Design review of the part built by this model. Coordinates are the model's own, in mm. A direction names the side the tool comes from. Coordinates: 2 decimals unless noted, no trailing zeros. Loops run counter-clockwise (first coordinate to the right, second up) from the corner with the lowest first, then second, coordinate; pieces in that order, holes last. Notation, with made-up numbers: (-27.5, 72.25) -> (24.5, 72.25) arc R24 ccw to (24.5, 82.25) -> close; hole circle Ø9 at (-6, 88). An arc over 180 degrees is marked (long way). Use a Markdown table: item, result. Add a question column.
Q1. For probe 1 along Y at (x, z) = (7, 0.4); probe 2 along Y at (x, z) = (9.5, 0.95); probe 3 along X at (y, z) = (7.25, 1.8), list the stretches that pass through material, from the lowest coordinate up.
Q2. Take a section at A-A on x = 9.5. Write out the cut boundary in (y, z), plus the area to 3 significant figures.
Q3. For faces 1 (the face through (11, 4, 1)), 2 (the face through (-4, 9, 1)), 3 (the face through (10, -7, 1)), 4 (the face through (8.95, 5.03, 1.08)), list the 3-axis set-ups (+Z, -Z, +X, -X, +Y, -Y) from which the entire face can be reached by the end or side of a thin tool; tool diameter is ignored.
Q4. Take a section at D-D on x = -1. Write out the cut boundary in (y, z).
Q5. Take a section at B-B on z = 1.4. Write out the cut boundary in (x, y).
Q6. Clearance check with flat-ended pins moving along their axes: pin 1 Ø1.1 at (x, z) = (8, 1) entering from +Y; pin 2 Ø1.1 at (y, z) = (8.5, 1.5) entering from -X; pin 3 Ø1.1 at (x, z) = (11, 1.5) entering from -Y. State where each tip first meets the part, or that it passes through.
Q7. Draft analysis for pull direction X (two halves, no side actions). For faces 5 (the face through (12.2, 0, 1)), 6 (the face through (8, 7.5, 1)), 7 (the face through (5.07, 6.45, 1.08)), state which applies: pulls with the +X half, pulls with the -X half, needs draft (parallel to the pull), parting line crosses it, or undercut.
Q8. Take a section at C-C on y = 1.25. Write out the cut boundary in (x, z).
from build123d import *

# Parameters (mm, degrees)
EXTRUDE_1_DEPTH = 2.2


with BuildPart() as part:
    # 草图1 → 凸台-拉伸1 (new body)
    with BuildSketch(Plane.XY):
        with BuildLine():
            Line((-4, 10.5), (-4, 7.5))
            ThreePointArc((-4, 7.5), (-5.05, 6.45), (-6.1, 7.5))
            Line((-6.1, 7.5), (-10, 7.5))
            Line((-10, 7.5), (-10, 5))
            Line((-10, 5), (6.666666667, -7.5))
            Line((6.666666667, -7.5), (10, -7.5))
            Line((10, -7.5), (10, -6.1))
            ThreePointArc((10, -6.1), (8.95, -5.05), (10, -4))
            Line((10, -4), (12.2, -4))
            Line((12.2, -4), (12.2, 4))
            Line((12.2, 4), (10, 4))
            ThreePointArc((10, 4), (8.95, 5.05), (10, 6.1))
            Line((10, 6.1), (10, 7.5))
            Line((10, 7.5), (6.1, 7.5))
            ThreePointArc((6.1, 7.5), (5.05, 6.45), (4, 7.5))
            Line((4, 7.5), (4, 10.5))
            Line((4, 10.5), (-4, 10.5))
        make_face()
    extrude(amount=EXTRUDE_1_DEPTH)


solid = part.part
Answer list:
| question | item | result |
|---|---|---|
| 1 | probe 1 | -7.5 to 7.5 |
| 1 | probe 2 | -7.5 to -5.97, -4.13 to 4.13, 5.97 to 7.5 |
| 1 | probe 3 | -10 to -6.07, -4.03 to 4.03, 6.07 to 10 |
| 2 | outline | (-7.5, 0) -> (-5.97, 0) -> (-5.97, 2.2) -> (-7.5, 2.2) -> close; (-4.13, 0) -> (4.13, 0) -> (4.13, 2.2) -> (-4.13, 2.2) -> close; (5.97, 0) -> (7.5, 0) -> (7.5, 2.2) -> (5.97, 2.2) -> close |
| 2 | area | 24.9 mm² |
| 3 | face 1 | +Z, -Z, +X, +Y |
| 3 | face 2 | +Z, -Z, -X, +Y |
| 3 | face 3 | +Z, -Z, +X, -Y |
| 3 | face 4 | +Z, -Z, +X |
| 4 | outline | (-1.75, 0) -> (10.5, 0) -> (10.5, 2.2) -> (-1.75, 2.2) -> close |
| 5 | outline | (-10, 5) -> (6.67, -7.5) -> (10, -7.5) -> (10, -6.1) arc R1.05 cw to (10, -4) -> (12.2, -4) -> (12.2, 4) -> (10, 4) arc R1.05 cw to (10, 6.1) -> (10, 7.5) -> (6.1, 7.5) arc R1.05 cw to (4, 7.5) -> (4, 10.5) -> (-4, 10.5) -> (-4, 7.5) arc R1.05 cw to (-6.1, 7.5) -> (-10, 7.5) -> close |
| 6 | pin 1 | y = 7.5 |
| 6 | pin 2 | x = -4 |
| 6 | pin 3 | y = -4 |
| 7 | face 5 | pulls with the +X half |
| 7 | face 6 | needs draft |
| 7 | face 7 | undercut |
| 8 | outline | (-5, 0) -> (12.2, 0) -> (12.2, 2.2) -> (-5, 2.2) -> close |
